from build123d import *

# Parameters (mm, degrees)
EXTRUDE_1_DEPTH     = 56
CUT_EXTRUDE_1_DEPTH = 56
SKETCH_3_R          = 2
CUT_EXTRUDE_2_DEPTH = 4
FILLET_1_R          = 2


with BuildPart() as part:
    # 草图1 → 凸台-拉伸1 (new body)
    with BuildSketch(Plane.XY):
        Polygon((0, 0), (37, 0), (37, 3), (3, 3), (3, 50), (0, 50), align=None)
    extrude(amount=EXTRUDE_1_DEPTH)

    # 草图2 → 切除-拉伸1 (cut)
    with BuildSketch(Plane(origin=(0, 3, 0), x_dir=(1, 0, 0), z_dir=(0, 1, 0))):
        with BuildLine():
            Line((11, -12.75), (31, -12.75))
            ThreePointArc((31, -12.75), (33.75, -10), (31, -7.25))
            Line((31, -7.25), (11, -7.25))
            ThreePointArc((11, -7.25), (8.25, -10), (11, -12.75))
        make_face()
        with BuildLine():
            Line((11, -43.25), (31, -43.25))
            ThreePointArc((31, -43.25), (33.75, -46), (31, -48.75))
            Line((31, -48.75), (11, -48.75))
            ThreePointArc((11, -48.75), (8.25, -46), (11, -43.25))
        make_face()
    extrude(amount=-CUT_EXTRUDE_1_DEPTH, mode=Mode.SUBTRACT)

    # 草图3 → 切除-拉伸2 (cut, through all)
    with BuildSketch(Plane(origin=(3, 0, 0), x_dir=(0, 0, -1), z_dir=(1, 0, 0))):
        with Locations((-52, 46)):
            Circle(SKETCH_3_R)
        with Locations((-4, 46)):
            Circle(SKETCH_3_R)
        with Locations((-4, 17.533468943)):
            Circle(SKETCH_3_R)
        with Locations((-52, 17.533468943)):
            Circle(SKETCH_3_R)
        with BuildLine():
            Line((-37, 41.766734471), (-19, 41.766734471))
            ThreePointArc((-19, 41.766734471), (-16.276373136, 41.388681089), (-13.758681543, 40.283105813))
            Line((-13.758681543, 40.283105813), (-11.678664761, 42.363122594))
            ThreePointArc((-11.678664761, 42.363122594), (-9.099000833, 42.363122594), (-9.099000833, 39.783458666))
            Line((-9.099000833, 39.783458666), (-11.049840185, 37.832619314))
            ThreePointArc((-11.049840185, 37.832619314), (-9, 31.766734471), (-11.049840185, 25.700849629))
            Line((-11.049840185, 25.700849629), (-9.099000833, 23.750010277))
            ThreePointArc((-9.099000833, 23.750010277), (-9.099000833, 21.170346349), (-11.678664761, 21.170346349))
            Line((-11.678664761, 21.170346349), (-13.758681543, 23.25036313))
            ThreePointArc((-13.758681543, 23.25036313), (-16.276373136, 22.144787854), (-19, 21.766734471))
            Line((-19, 21.766734471), (-37, 21.766734471))
            ThreePointArc((-37, 21.766734471), (-39.723626864, 22.144787854), (-42.241318457, 23.25036313))
            Line((-42.241318457, 23.25036313), (-44.321335239, 21.170346349))
            ThreePointArc((-44.321335239, 21.170346349), (-46.900999167, 21.170346349), (-46.900999167, 23.750010277))
            Line((-46.900999167, 23.750010277), (-44.950159815, 25.700849629))
            ThreePointArc((-44.950159815, 25.700849629), (-47, 31.766734471), (-44.950159815, 37.832619314))
            Line((-44.950159815, 37.832619314), (-46.900999167, 39.783458666))
            ThreePointArc((-46.900999167, 39.783458666), (-46.900999167, 42.363122594), (-44.321335239, 42.363122594))
            Line((-44.321335239, 42.363122594), (-42.241318457, 40.283105813))
            ThreePointArc((-42.241318457, 40.283105813), (-39.723626864, 41.388681089), (-37, 41.766734471))
        make_face()
    extrude(amount=-CUT_EXTRUDE_2_DEPTH, mode=Mode.SUBTRACT)

    # 圆角1
    fillet_1_edges = [part.edges().sort_by_distance(p)[0] for p in [
        (37, 1.5, 56),
        (0, 0, 28),
        (1.5, 50, 56),
        (1.5, 50, 0),
        (37, 1.5, 0),
    ]]
    fillet(fillet_1_edges, radius=FILLET_1_R)


solid = part.part
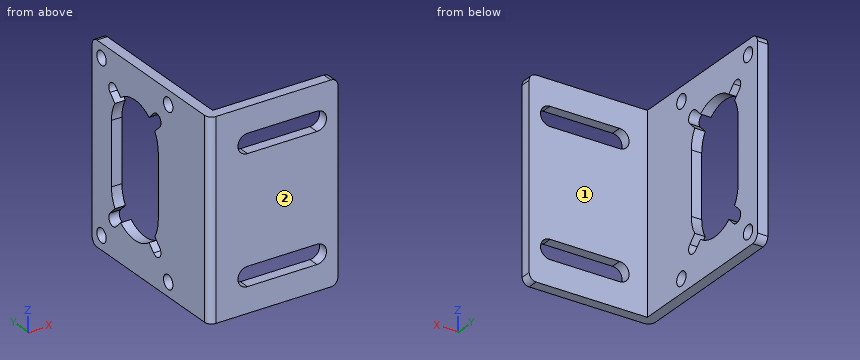
The listing builds one solid part. Answer for the finished solid, in the listing's coordinates (mm). Face numbers are marked on the shaded views. A direction names the side the tool comes from. Coordinates: 2 decimals unless noted, no trailing zeros. Write each loop counter-clockwise with the first axis right and the second up, starting at its lowest first coordinate (ties: lowest second). Pieces come first, ordered by that corner, then holes. Notation, with made-up numbers: (-38, -21.75) - (-33, -21.75) arc R29 cw to (-33, 11.25) - close; hole circle Ø10 at (20.25, -24). An arc over 180 degrees is marked (long way). Answer as CSV lines item,"result".
1. Straight lines are drawn through the part: line 1 (Y direction, x = 2.05, z = 4); line 2 (Y direction, x = 0.8, z = 4); line 3 (Y direction, x = 31.5, z = 2.5). For each, find the intervals that lie inside material, in ascending order. Write a range as [from, to].
Computed values:
line 1,"y = [0, 15.53], [19.53, 44], [48, 50]"
line 2,"y = [0.4, 15.53], [19.53, 44], [48, 50]"
line 3,"y = [0, 3]"
2. Find section C-C (z = 26). Give the vertices of the cut face in (x, y), plus the area to 3 significant figures.
Computed values:
outline,"(0, 2) arc R2 ccw to (2, 0) - (37, 0) - (37, 3) - (3, 3) - (3, 21.77) - (0, 21.77) - close; (0, 41.77) - (3, 41.77) - (3, 50) - (0, 50) - close"
area,"191 mm²"
3. Find section D-D (z = 4). Give the vertices of the cut face in (x, y), plus the area to 3 significant figures.
Computed values:
outline,"(0, 2) arc R2 ccw to (2, 0) - (37, 0) - (37, 3) - (3, 3) - (3, 15.53) - (0, 15.53) - close; (0, 19.53) - (3, 19.53) - (3, 44) - (0, 44) - close; (0, 48) - (3, 48) - (3, 50) - (0, 50) - close"
area,"227 mm²"
4. Find section A-A (x = 26). Give the vertices of the cut face in (y, z).
Computed values:
outline,"(0, 0) - (3, 0) - (3, 7.25) - (0, 7.25) - close; (0, 12.75) - (3, 12.75) - (3, 43.25) - (0, 43.25) - close; (0, 48.75) - (3, 48.75) - (3, 56) - (0, 56) - close"
5. Find section B-B (y = 46). Give the vertices of the cut face in (x, z).
Computed values:
outline,"(0, 0) - (3, 0) - (3, 2) - (0, 2) - close; (0, 6) - (3, 6) - (3, 50) - (0, 50) - close; (0, 54) - (3, 54) - (3, 56) - (0, 56) - close"
6. Given P1, Ø3, axis at y = 38.5, z = 47, coming from the -X side; P2, Ø5, axis at y = 46, z = 52, coming from the +X side; P3, Ø5, axis at x = 18, z = 13, coming from the +Y side; P4, Ø3.5, axis at y = 17.53, z = 52, coming from the +X side, each flat-ended and moving along its own axis, determine where each tip first touches the part or whether it passes through.
Computed values:
P1,"stops at x = 0"
P2,"stops at x = 3"
P3,"stops at y = 3"
P4,"passes through"
7. A tool of negligible diameter and unlimited length cuts with its end or side. For the marked faces 1 and 2, from which of +Z, -Z, +X, -X, +Y, -Y can it reach the whole face along a straight path? Write none if from no direction.
Computed values:
face 1,"+Z, -Z, +X, +Y"
face 2,"+Z, -Z, +X, -X, -Y"
